Source: CAD feature listing. Evaluate the final solid. Frame: model axes, mm. A direction names the side the tool comes from. Round coordinates to 2 decimals unless told otherwise and drop trailing zeros. Order: outer loops, then holes, each group sorted by start corner. A loop starts at its lowest first (then second) coordinate and runs counter-clockwise, first axis right, second up. Notation, with made-up numbers: M 83.5,87 L 137.5,87 A8 cw 137.5,93 Z; hole C 45,-27.75 d6. An arc over 180 degrees is marked long. Answer in a Markdown table with one row per item. Add a question column.
```python
from build123d import *

# Parameters (mm, degrees)
F1_DEPTH  = 60
F3_DEPTH  = 15
F5_DEPTH  = 15.001
F7_DEPTH  = 15.001
F9_DEPTH  = 60.001
F11_REACH = 66.0565127546
F12_R     = 9.999


# Not quite as in the source:
# - a fillet or chamfer is up to 0.001 mm smaller than in the source, because OpenCascade refuses the exact size


with BuildPart() as f1:
    # F0 (on Front) → F1 (new body)
    with BuildSketch(Plane.XZ):
        with BuildLine():
            Line((-30, 0), (30, 0))
            ThreePointArc((30, 0), (0, 30), (-30, 0))
        make_face()
    extrude(amount=F1_DEPTH)

    # F2 (on face) → F3 (join)
    with BuildSketch(Plane(origin=(0, 0, 0), x_dir=(1, 0, 0), z_dir=(0, 0, -1))):
        with BuildLine():
            ThreePointArc((-40, 20), (-50, 10), (-40, 0))
            Line((-40, 0), (40, 0))
            ThreePointArc((40, 0), (50, 10), (40, 20))
            Line((40, 20), (-40, 20))
        make_face()
    extrude(amount=-F3_DEPTH)

    # F4 (on face) → F5 (cut, through all)
    with BuildSketch(Plane.XY.offset(15)):
        with BuildLine():
            Line((-45, -10), (-40, -10))
            Line((-40, -10), (-40, -5))
            ThreePointArc((-40, -5), (-43.5355339059, -6.4644660941), (-45, -10))
        make_face()
        with BuildLine():
            Line((-40, -5), (-40, -10))
            Line((-40, -10), (-35, -10))
            ThreePointArc((-35, -10), (-36.4644660941, -6.4644660941), (-40, -5))
        make_face()
        with BuildLine():
            Line((-40, -10), (-40, -15))
            ThreePointArc((-40, -15), (-36.4644660941, -13.5355339059), (-35, -10))
            Line((-35, -10), (-40, -10))
        make_face()
        with BuildLine():
            ThreePointArc((-45, -10), (-43.5355339059, -13.5355339059), (-40, -15))
            Line((-40, -15), (-40, -10))
            Line((-40, -10), (-45, -10))
        make_face()
    extrude(amount=-F5_DEPTH, mode=Mode.SUBTRACT)

    # F6 (on face) → F7 (cut, through all)
    with BuildSketch(Plane.XY.offset(15)):
        with BuildLine():
            ThreePointArc((40, -5), (36.4644660941, -6.4644660941), (35, -10))
            Line((35, -10), (40, -10))
            Line((40, -10), (40, -5))
        make_face()
        with BuildLine():
            Line((40, -5), (40, -10))
            Line((40, -10), (45, -10))
            ThreePointArc((45, -10), (43.5355339059, -6.4644660941), (40, -5))
        make_face()
        with BuildLine():
            Line((45, -10), (40, -10))
            Line((40, -10), (40, -15))
            ThreePointArc((40, -15), (43.5355339059, -13.5355339059), (45, -10))
        make_face()
        with BuildLine():
            Line((40, -10), (35, -10))
            ThreePointArc((35, -10), (36.4644660941, -13.5355339059), (40, -15))
            Line((40, -15), (40, -10))
        make_face()
    extrude(amount=-F7_DEPTH, mode=Mode.SUBTRACT)

    # F8 (on face) → F9 (cut, through all)
    with BuildSketch(Plane.XZ.offset(60)):
        with BuildLine():
            Line((-25, 0), (25, 0))
            ThreePointArc((25, 0), (0, 25), (-25, 0))
        make_face()
    extrude(amount=-F9_DEPTH, mode=Mode.SUBTRACT)

    f11_end = f1.faces().sort_by_distance((0, -30, 30))[0]
    # F10 (on Top) → F11 (cut, up to a face of the model that its end follows)
    with BuildSketch(Plane.XY):
        Polygon((-10, -60), (0, -60), (10, -60), (10, -30), (-10, -30), align=None)
    f11_long = extrude(amount=F11_REACH, mode=Mode.PRIVATE)
    add(split(f11_long, bisect_by=f11_end, keep=Keep.BOTTOM, mode=Mode.PRIVATE), mode=Mode.SUBTRACT)

    # F12 (radius 10 in the source; OpenCascade refuses exactly that, so slightly less here)
    f12_edges = [f1.edges().sort_by_distance(p)[0] for p in [
        (-10, -30, 25.598575),
        (10, -30, 25.598575),
    ]]
    fillet(f12_edges, radius=F12_R)


solid = f1.part
```
(1) Pin query (flat end, axial travel): pin 1 (16 mm diameter, centred on x = -43.5, y = -11, fed in from +Z); pin 2 (1.6 mm diameter, centred on y = -49.5, z = 26.5, fed in from +X); pin 3 (4.5 mm diameter, centred on y = -52.5, z = 25, fed in from -X). Return the tip coordinate at first contact, or that it passes through.
(2) Cut plane B-B (y = -37.5). Return loops of the section in (x, z), and give its area (3 significant figures).
(3) Draft query along X for faces 1 (the face through (-10, -50, 26)), 2 (the face through (21, -60, 15)), 3 (the face through (-50, -10, 7)). Return one class per face: +X half, -X half, draft (parallel to the pull), parting line (faces both ways), or undercut.
(4) Line query: line 1 (Y direction, x = -30, z = 6); line 2 (X direction, y = -9, z = 3); line 3 (X direction, y = -37.5, z = 23). Output: solid intervals per line, ascending. Write a range as from..to.
(5) Access query for faces 4 (the face through (-34, -20, 7)), 5 (the face through (-7.15, -33.01, 26.51)), 6 (the face through (0.66, -29.58, 29.993)). Directions: +Z, -Z, +X, -X, +Y, -Y. A direction counts if a zero-diameter tool reaches every point of the face in a straight line with its end or side. Return the directions, or none.
(6) Cut plane D-D (z = 8). Return loops of the section in (x, y).
(7) Cut plane A-A (z = 2.5). Return loops of the section in (x, y), and give its area (3 significant figures).
(8) Cut plane C-C (z = 24). Return loops of the section in (x, y).
Answer list:
| question | item | result |
|---|---|---|
| 1 | pin 1 | z = 15 |
| 1 | pin 2 | x = 15.48 |
| 1 | pin 3 | x = -19.56 |
| 2 | outline | M -30,0 L -25,0 A25 cw -9.68,23.05 L -9.68,28.39 A30 ccw Z; M 9.68,23.05 A25 cw 25,0 L 30,0 A30 ccw 9.68,28.39 Z |
| 2 | area | 333 mm² |
| 3 | face 1 | undercut |
| 3 | face 2 | draft |
| 3 | face 3 | -X half |
| 4 | line 1 | -20..0 |
| 4 | line 2 | -49.95..-44.9, -35.1..-24.82, 24.82..35.1, 44.9..49.95 |
| 4 | line 3 | -19.26..-9.8, 9.8..19.26 |
| 5 | face 4 | +Z, -X, -Y |
| 5 | face 5 | +Z, -Z, -Y |
| 5 | face 6 | +Z, -Y |
| 6 | outline | M -40,-20 L -28.91,-20 L -28.91,-60 L -23.69,-60 L -23.69,0 L -40,0 A10 ccw Z; M 23.69,-60 L 28.91,-60 L 28.91,-20 L 40,-20 A10 ccw 40,0 L 23.69,0 Z; hole C -40,-10 d10; hole C 40,-10 d10 |
| 7 | outline | M -40,-20 L -29.9,-20 L -29.9,-60 L -24.87,-60 L -24.87,0 L -40,0 A10 ccw Z; M 24.87,-60 L 29.9,-60 L 29.9,-20 L 40,-20 A10 ccw 40,0 L 24.87,0 Z; hole C -40,-10 d10; hole C 40,-10 d10 |
| 7 | area | 1,160 mm² |
| 8 | outline | M -18,-60 L -10,-60 L -10,-40 A10 cw -7,-32.86 L -7,0 L -18,0 Z; M 7,-32.86 A10 cw 10,-40 L 10,-60 L 18,-60 L 18,0 L 7,0 Z |
